Verification items for this drawing (mm, ordinates from the low corner). Coordinates: 2 decimals unless noted, no trailing zeros. Order: outer loops, then holes, each group sorted by start corner. A loop starts at its lowest first (then second) coordinate and runs counter-clockwise, first axis right, second up. Notation, with made-up numbers: M 38,-10.75 L 83,-10.75 A26 cw 83,7.25 Z; hole C 13.25,-38.75 d7. An arc over 180 degrees is marked long. Use CSV: the item, a comma, the result in double quotes. Start each with the question number.
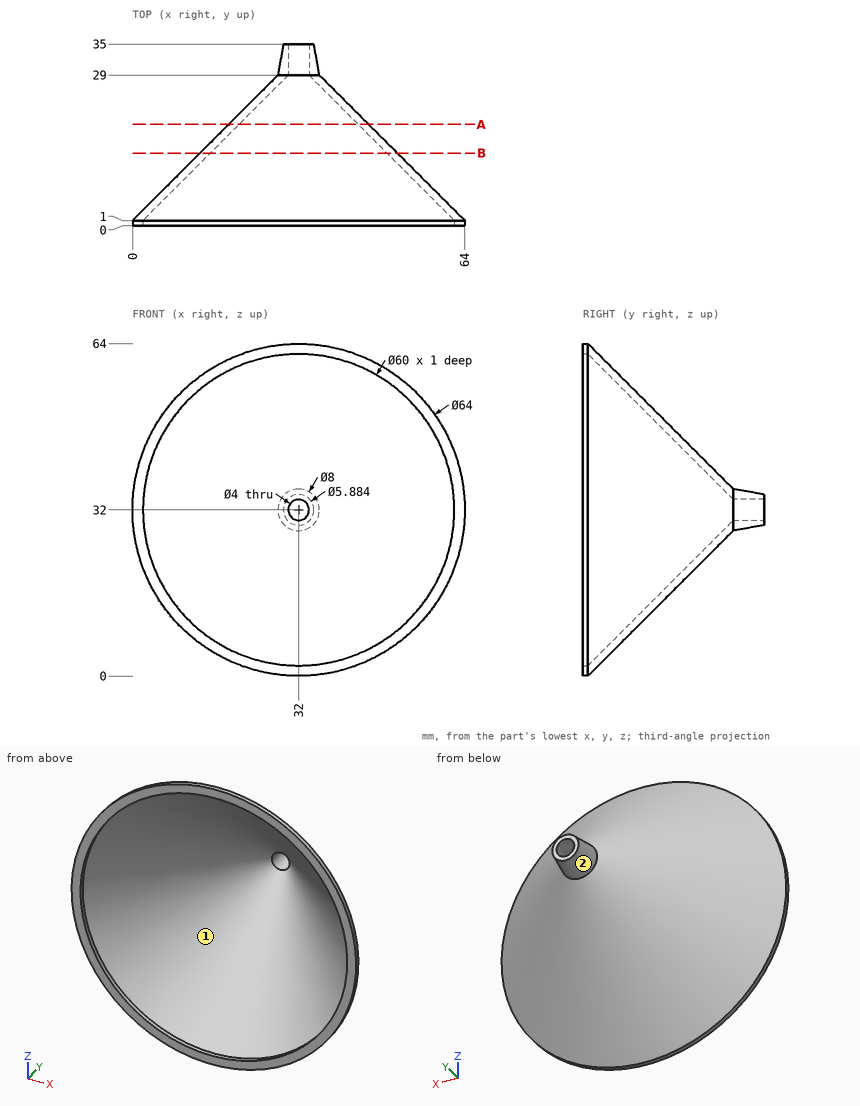
1) Gauge pin test, flat ends, axial feed: P1, Ø1, axis at x = 48, z = 18, coming from the +Y side; P2, Ø3, axis at x = 27.5, y = 20.5, coming from the -Z side; P3, Ø6, axis at y = 7, z = 20.5, coming from the +X side; P4, Ø2.5, axis at x = 32, z = 32, coming from the -Y side. Record the tip position at first contact, or that the pin passes through.
2) Section check B-B on y = 14. Record the boundary of the cut face in (x, z), then the cut area to 3 significant figures.
3) Section check A-A on y = 19.5. Record the boundary of the cut face in (x, z), then the cut area to 3 significant figures.
4) Material ranges on line 1 along X through (y, z) = (0.3, 32); line 2 along X through (y, z) = (10.5, 16); line 3 along Z through (x, y) = (21.5, 12.5), recorded low to high.
5) Draft check along Z on the marked faces 1 and 2. Enter one of: +Z half, -Z half, draft (parallel to the pull), parting line (faces both ways), or undercut.
Results are:
1,P1,"stops at y = 12.24"
1,P2,"stops at z = 18.67"
1,P3,"stops at x = 58.85"
1,P4,"passes through"
2,outline,"C 32,32 d38; hole C 32,32 d34"
2,area,"226 mm²"
3,outline,"C 32,32 d27; hole C 32,32 d23"
3,area,"157 mm²"
4,line 1,"x = 0 to 2, 62 to 64"
4,line 2,"x = 16.18 to 19.18, 44.82 to 47.82"
4,line 3,"z = 14.39 to 16.77, 47.23 to 49.61"
5,face 1,"undercut"
5,face 2,"parting line"
